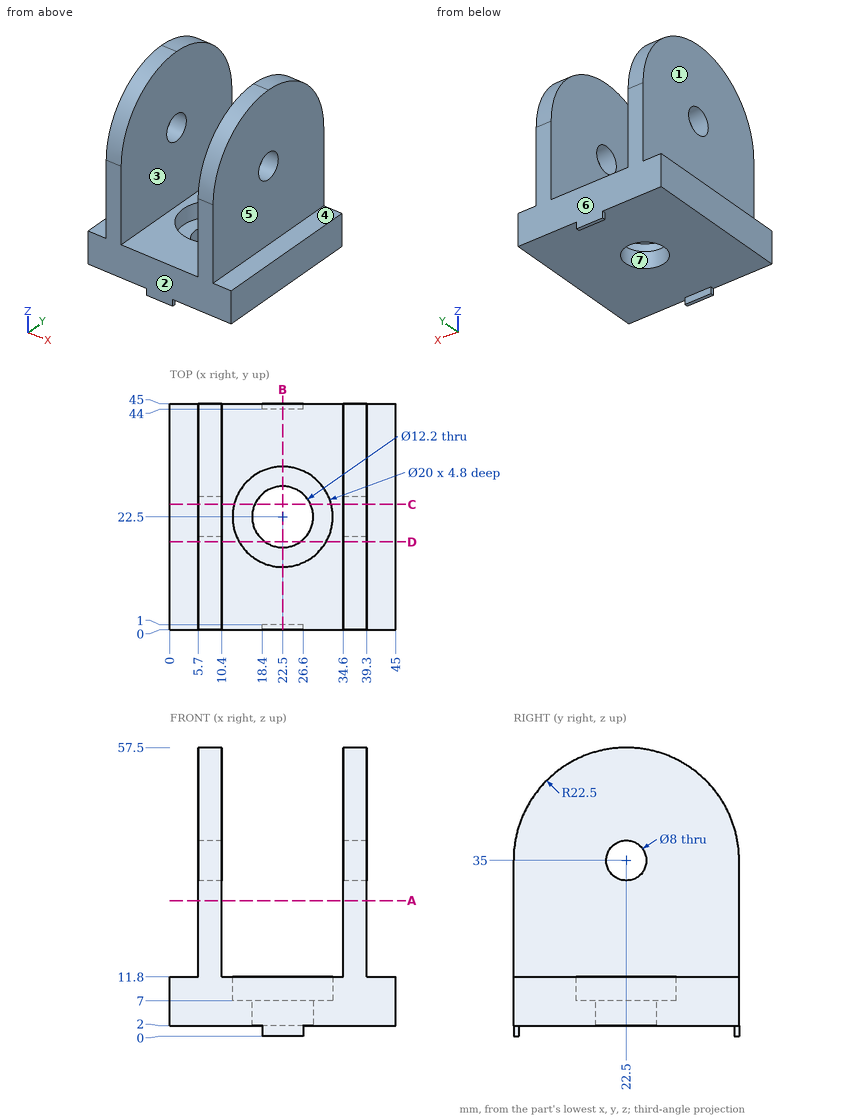
Here's the drawing with two shaded views (mm, measured from the low corner). I have some questions. A direction names the side the tool comes from. Give positions to 0.01 mm unless a question says otherwise; leave off trailing zeros. Loops run counter-clockwise (first coordinate to the right, second up) from the corner with the lowest first, then second, coordinate; pieces in that order, holes last. Notation, with made-up numbers: (66.25, 21) - (91.25, 21) arc R16 cw to (91.25, 45) - close; hole circle Ø2 at (57, 26). An arc over 180 degrees is marked (long way). Return JSON: item names as keys, results as strings.
1. I'm going to push flat-ended pins straight in: pin 1 Ø1.5 at (y, z) = (15, 41.5) entering from +X; pin 2 Ø6.5 at (x, y) = (42, 17.5) entering from +Z; pin 3 Ø16 at (x, y) = (22.5, 22.5) entering from +Z. Where does each tip first touch, or does it pass through?
Output values:
{"pin 1": "stops at x = 39.3", "pin 2": "stops at z = 57.27", "pin 3": "stops at z = 7"}
2. If I drill on line 1 (X direction, y = 32.5, z = 13); line 2 (Y direction, x = 22.5, z = 8.7); line 3 (Z direction, x = 28.5, y = 42), over which ranges is the centre line in solid material (lowest first)?
Output values:
{"line 1": "x = 5.7 to 10.4, 34.6 to 39.3", "line 2": "y = 0 to 12.5, 32.5 to 45", "line 3": "z = 2 to 11.8"}
3. For the marked faces 1, 2, 3 and 4, which set-ups out of +Z, -Z, +X, -X, +Y, -Y let a thin tool reach every point of the face, with its end or its side?
Output values:
{"face 1": "+Z, -X, +Y, -Y", "face 2": "+Z, -Z, +X, -X, -Y", "face 3": "+Z, +Y, -Y", "face 4": "+Z, +X, +Y, -Y"}
4. I want a section at A-A on z = 27. Please give me the cut outline in (x, y).
Output values:
{"outline": "(5.7, 0) - (10.4, 0) - (10.4, 45) - (5.7, 45) - close; (34.6, 0) - (39.3, 0) - (39.3, 45) - (34.6, 45) - close"}
5. We'd pull the mould along Y, two halves only. Please class the marked faces 5, 6 and 7: +Y half, -Y half, draft (parallel to the pull), parting line (faces both ways), or undercut.
Output values:
{"face 5": "draft", "face 6": "+Y half", "face 7": "undercut"}
6. I want a section at B-B on x = 22.5. Please give me the cut outline in (y, z), and give its area (3 significant figures).
Output values:
{"outline": "(0, 0) - (1, 0) - (1, 2) - (16.4, 2) - (16.4, 7) - (12.5, 7) - (12.5, 11.8) - (0, 11.8) - close; (28.6, 2) - (44, 2) - (44, 0) - (45, 0) - (45, 11.8) - (32.5, 11.8) - (32.5, 7) - (28.6, 7) - close", "area": "288 mm²"}
7. I want a section at C-C on y = 25. Please give me the cut outline in (x, z), and give its area (3 significant figures).
Output values:
{"outline": "(0, 2) - (16.94, 2) - (16.94, 7) - (12.82, 7) - (12.82, 11.8) - (10.4, 11.8) - (10.4, 31.88) - (5.7, 31.88) - (5.7, 11.8) - (0, 11.8) - close; (5.7, 38.12) - (10.4, 38.12) - (10.4, 57.36) - (5.7, 57.36) - close; (28.06, 2) - (45, 2) - (45, 11.8) - (39.3, 11.8) - (39.3, 31.88) - (34.6, 31.88) - (34.6, 11.8) - (32.18, 11.8) - (32.18, 7) - (28.06, 7) - close; (34.6, 38.12) - (39.3, 38.12) - (39.3, 57.36) - (34.6, 57.36) - close", "area": "662 mm²"}
8. I want a section at D-D on y = 17.5. Please give me the cut outline in (x, z), and give its area (3 significant figures).
Output values:
{"outline": "(0, 2) - (19.01, 2) - (19.01, 7) - (13.84, 7) - (13.84, 11.8) - (10.4, 11.8) - (10.4, 56.94) - (5.7, 56.94) - (5.7, 11.8) - (0, 11.8) - close; (25.99, 2) - (45, 2) - (45, 11.8) - (39.3, 11.8) - (39.3, 56.94) - (34.6, 56.94) - (34.6, 11.8) - (31.16, 11.8) - (31.16, 7) - (25.99, 7) - close", "area": "747 mm²"}
